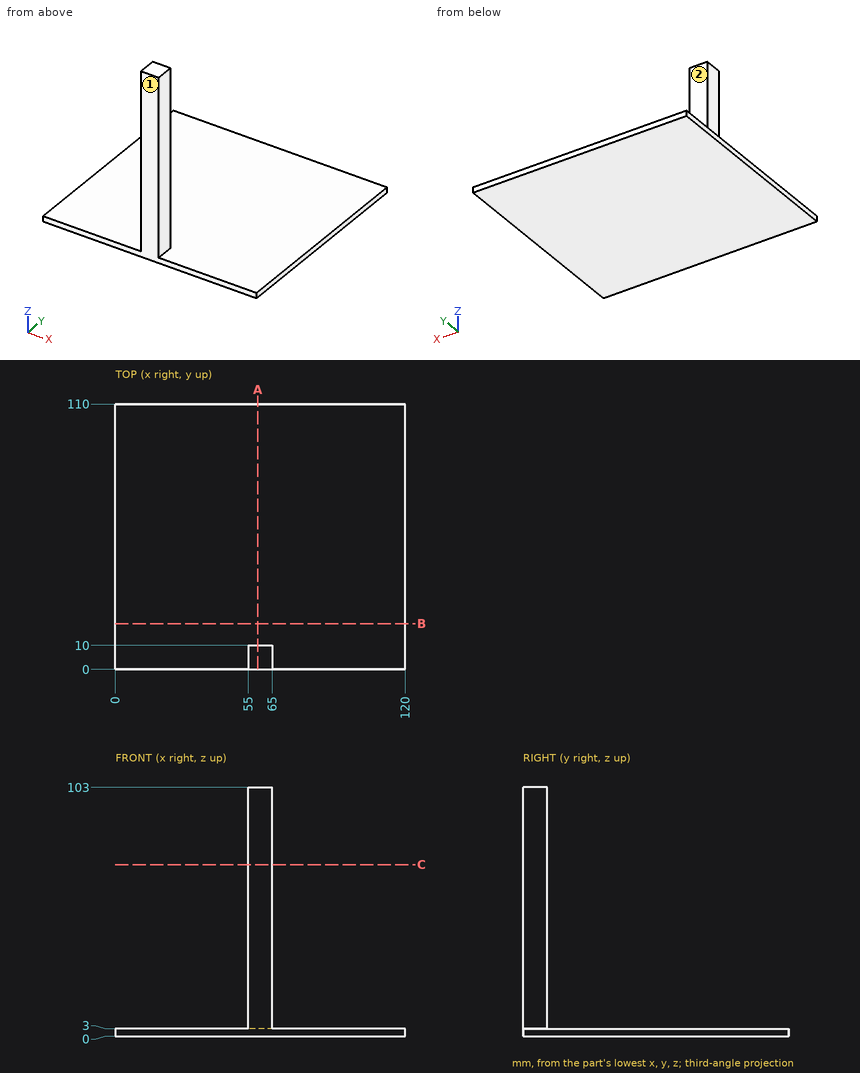
Could you check a few things on this drawing? It's one solid part, dimensions in mm from its lowest x, y, z. A direction names the side the tool comes from. Coordinates: 2 decimals unless noted, no trailing zeros. Write each loop counter-clockwise with the first axis right and the second up, starting at its lowest first coordinate (ties: lowest second). Pieces come first, ordered by that corner, then holes. Notation, with made-up numbers: M -6,87.5 L 47,87.5 A13 ccw 47,100.5 Z; hole C -11,13 d3. An arc over 180 degrees is marked long. One line per question, with ' | ' between items.
1) Imagine slicing it at C-C, the plane z = 71. Write out the boundary of the cut face in (x, y).
Checks:
outline: M 55,0 L 65,0 L 65,10 L 55,10 Z
2) For the marked faces 1 and 2, which set-ups out of +Z, -Z, +X, -X, +Y, -Y let a thin tool reach every point of the face, with its end or its side?
Checks:
face 1: +Z, -Z, +X, -X, -Y | face 2: +Z, +X, -X, +Y
3) Imagine slicing it at A-A, the plane x = 59. Write out the boundary of the cut face in (y, z).
Checks:
outline: M 0,0 L 110,0 L 110,3 L 10,3 L 10,103 L 0,103 Z
4) For pin 1 Ø1 at (x, y) = (49.5, 89) entering from -Z; pin 2 Ø11 at (y, z) = (3.5, 35.5) entering from -X; pin 3 Ø5 at (y, z) = (2.5, 36) entering from +X; pin 4 Ø2 at (x, y) = (77, 65.5) entering from +Z, each with a flat end and sliding along its axis, tell me the tip position at first contact or that it passes through.
Checks:
pin 1: z = 0 | pin 2: x = 55 | pin 3: x = 65 | pin 4: z = 3
5) I need wall thicknesses on probe 1 along Z at (x, y) = (54.5, 57); probe 2 along Y at (x, z) = (56, 58.5); probe 3 along X at (y, z) = (7, 49.5). Which ranges of each line are inside material? Lowest first, please. Write a range as [from, to].
Checks:
probe 1: [0, 3] | probe 2: [0, 10] | probe 3: [55, 65]
6) Imagine slicing it at B-B, the plane y = 19. Write out the boundary of the cut face in (x, z), and give its area (3 significant figures).
Checks:
outline: M 0,0 L 120,0 L 120,3 L 0,3 Z | area: 360 mm²
